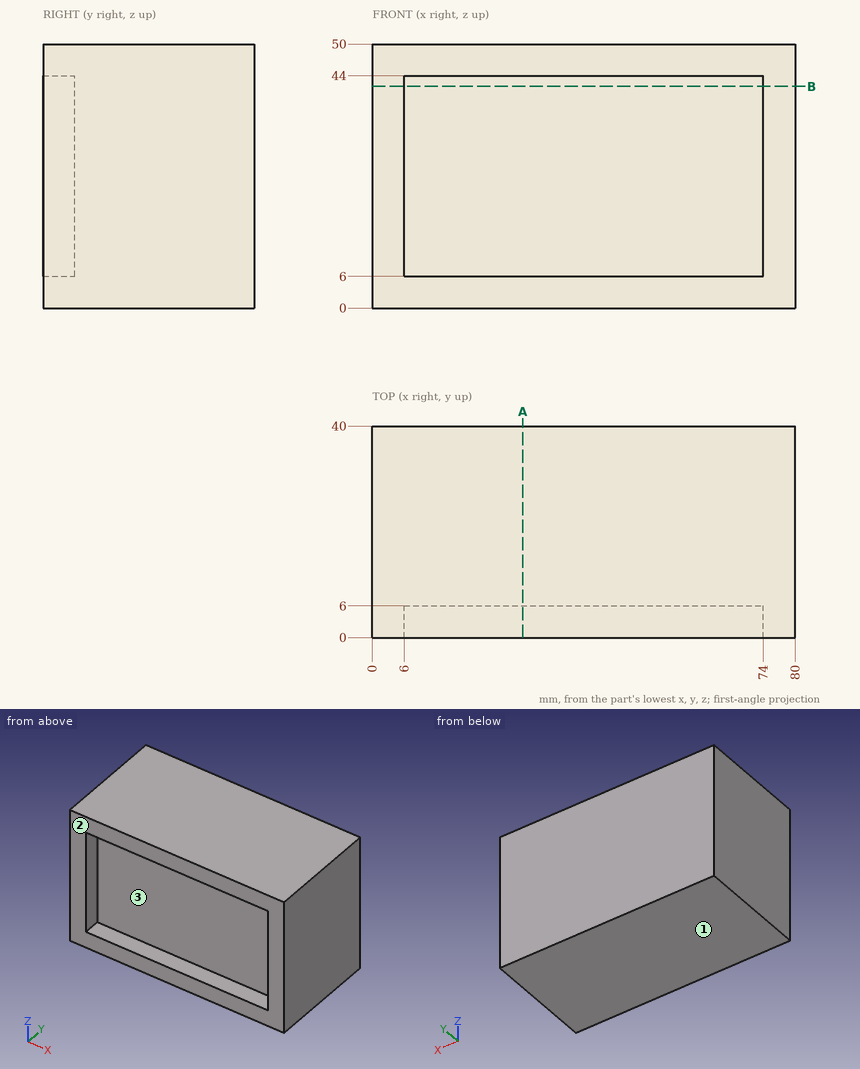
For this review, use the dimensioned drawing (mm, ordinates from the lowest corner) and the shaded views. Round coordinates to 2 decimals unless told otherwise and drop trailing zeros. Write each loop counter-clockwise with the first axis right and the second up, starting at its lowest first coordinate (ties: lowest second). Pieces come first, ordered by that corner, then holes. Notation, with made-up numbers: (57.5, 24) -> (79.5, 24) arc R10 cw to (79.5, 32) -> close; hole circle Ø10 at (63, 38). An arc over 180 degrees is marked (long way). Use CSV: the item, a comma, the result in double quotes.
(1) Draft analysis for pull direction Z (two halves, no side actions). For the marked faces 1, 2 and 3, state which applies: +Z half, -Z half, draft (parallel to the pull), parting line (faces both ways), or undercut.
Computed values:
face 1,"-Z half"
face 2,"draft"
face 3,"undercut"
(2) Consider section B-B, the plane z = 42. Give the boundary of the cut face in (x, y), plus the area to 3 significant figures.
Computed values:
outline,"(0, 0) -> (6, 0) -> (6, 6) -> (74, 6) -> (74, 0) -> (80, 0) -> (80, 40) -> (0, 40) -> close"
area,"2,790 mm²"
(3) To check wall thickness, follow L1, parallel to Z at x = 16, y = 3; L2, parallel to Y at x = 48.5, z = 20.5. State the ranges of each line that lie inside material, in increasing order. Write a range as [from, to].
Computed values:
L1,"[0, 6], [44, 50]"
L2,"[6, 40]"
(4) Clearance check with a flat-ended pin moving along its axis: P1, Ø19, axis at x = 48.5, z = 24, coming from the -Y side. State where the tip first meets the part, or that it passes through.
Computed values:
P1,"y = 6"
(5) Consider section A-A, the plane x = 28.5. Give the boundary of the cut face in (y, z).
Computed values:
outline,"(0, 0) -> (40, 0) -> (40, 50) -> (0, 50) -> (0, 44) -> (6, 44) -> (6, 6) -> (0, 6) -> close"
